Here's how the part is built. I have some questions about the finished solid (model axes, mm). Round coordinates to 2 decimals unless told otherwise and drop trailing zeros. Loops run counter-clockwise (first coordinate to the right, second up) from the corner with the lowest first, then second, coordinate; pieces in that order, holes last. Notation, with made-up numbers: M 10.5,70.5 L 38.5,70.5 A19 ccw 38.5,93.5 Z; hole C -9.5,-27.5 d2. An arc over 180 degrees is marked long. Answer as CSV lines item,"result".
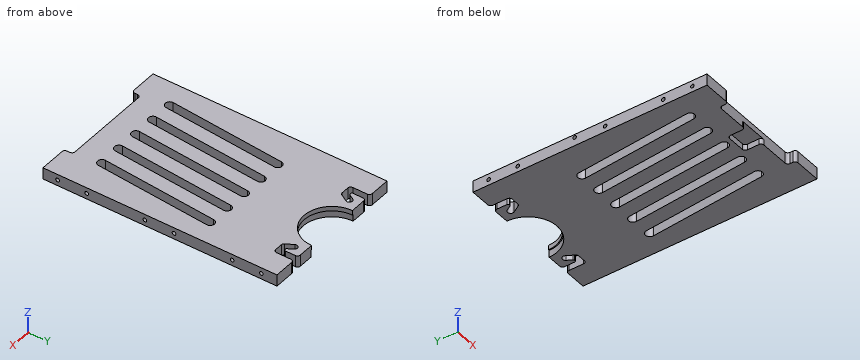
```python
from build123d import *

# Parameters (mm, degrees)
SKETCH1_W                       = 165.1
SKETCH1_H                       = 12.7
BOSS_EXTRUDE1_DEPTH             = 128.5875
SKETCH2_R                       = 30.63494
CUT_EXTRUDE1_DEPTH              = 154.33146336
SKETCH3_R                       = 31.75
CUT_EXTRUDE2_DEPTH              = 7.62
CUT_EXTRUDE3_DEPTH              = 154.33146336
FILLET1_R                       = 3.175
FILLET2_R                       = 1.5875
SKETCH5_W                       = 101.6
SKETCH5_H                       = 9.525
CUT_EXTRUDE4_DEPTH              = 154.33146336
FILLET3_R                       = 3.175
F_21_0_159_DIAMETER_HOLE2_D     = 4.0386
F_21_0_159_DIAMETER_HOLE2_DEPTH = 20.6375
F_21_0_159_DIAMETER_HOLE2_TIP   = 1.213317848
CUT_EXTRUDE5_DEPTH              = 154.33146336
SKETCH11_W                      = 25.4
SKETCH11_H                      = 19.05
CUT_EXTRUDE6_DEPTH              = 6.35
FILLET4_R                       = 3.175


# Read off the part's stored shape, not the designer's step: #21 (0.159) Diameter Hole1
with BuildPart() as part:
    # Sketch1 → Boss-Extrude1 (new, symmetric)
    with BuildSketch(Plane(origin=(0, 0, 0), x_dir=(1, 0, 0), z_dir=(0, 1, 0))):
        Rectangle(SKETCH1_W, SKETCH1_H)
    extrude(amount=BOSS_EXTRUDE1_DEPTH, both=True)

    # Sketch2 → Cut-Extrude1 (cut, through all)
    with BuildSketch(Plane.XY.offset(6.35)):
        with Locations((0, 128.5875)):
            Circle(SKETCH2_R)
    extrude(amount=-CUT_EXTRUDE1_DEPTH, mode=Mode.SUBTRACT)

    # Sketch3 → Cut-Extrude2 (cut)
    with BuildSketch(Plane(origin=(0, 0, -6.35), x_dir=(-1, 0, 0), z_dir=(0, 0, -1))):
        with Locations((0, 128.5875)):
            Circle(SKETCH3_R)
    extrude(amount=-CUT_EXTRUDE2_DEPTH, mode=Mode.SUBTRACT)

    # Sketch4 → Cut-Extrude3 (cut, through all)
    with BuildSketch(Plane.XY.offset(6.35)):
        with BuildLine():
            Line((57.277, 128.5875), (57.277, 106.3625))
            Line((57.277, 106.3625), (43.877983689, 106.3625))
            Line((43.877983689, 106.3625), (38.415384653, 115.823999072))
            ThreePointArc((38.415384653, 115.823999072), (39.623999536, 120.334615615), (44.134615883, 119.126))
            Line((44.134615883, 119.126), (47.690804866, 112.9665))
            Line((47.690804866, 112.9665), (50.673, 112.9665))
            Line((50.673, 112.9665), (50.673, 128.5875))
            Line((50.673, 128.5875), (57.277, 128.5875))
        make_face()
        with BuildLine():
            Line((-50.673, 128.5875), (-57.277, 128.5875))
            Line((-57.277, 128.5875), (-57.277, 106.3625))
            Line((-57.277, 106.3625), (-43.877983689, 106.3625))
            Line((-43.877983689, 106.3625), (-38.415384653, 115.823999072))
            ThreePointArc((-38.415384653, 115.823999072), (-39.623999536, 120.334615615), (-44.134615883, 119.126))
            Line((-44.134615883, 119.126), (-47.690804866, 112.9665))
            Line((-47.690804866, 112.9665), (-50.673, 112.9665))
            Line((-50.673, 112.9665), (-50.673, 128.5875))
        make_face()
    extrude(amount=-CUT_EXTRUDE3_DEPTH, mode=Mode.SUBTRACT)

    # Fillet1
    fillet1_edges = [part.edges().sort_by_distance(p)[0] for p in [
        (50.673, 128.5875, 0),
        (57.277, 128.5875, 0),
        (57.277, 106.3625, 0),
        (43.877983689, 106.3625, 0),
        (-43.877983689, 106.3625, 0),
        (-57.277, 106.3625, 0),
        (-57.277, 128.5875, 0),
        (-50.673, 128.5875, 0),
    ]]
    fillet(fillet1_edges, radius=FILLET1_R)

    # Fillet2
    fillet2_edges = [part.edges().sort_by_distance(p)[0] for p in [
        (47.690804866, 112.9665, 0),
        (50.673, 112.9665, 0),
        (-50.673, 112.9665, 0),
        (-47.690804866, 112.9665, 0),
    ]]
    fillet(fillet2_edges, radius=FILLET2_R)

    # Sketch5 → Cut-Extrude4 (cut, through all)
    with BuildSketch(Plane.XY.offset(6.35)):
        with Locations((0, -123.825)):
            Rectangle(SKETCH5_W, SKETCH5_H)
    extrude(amount=-CUT_EXTRUDE4_DEPTH, mode=Mode.SUBTRACT)

    # Fillet3
    fillet3_edges = [part.edges().sort_by_distance(p)[0] for p in [
        (-50.8, -128.5875, 0),
        (-50.8, -119.0625, 0),
        (50.8, -119.0625, 0),
        (50.8, -128.5875, 0),
    ]]
    fillet(fillet3_edges, radius=FILLET3_R)

    # #21 (0.159) Diameter Hole1 outline → #21 (0.159) Diameter Hole1 (revolve, cut)
    with BuildSketch(Plane(origin=(0, 111.41250006, 0), x_dir=(0, 1, 0), z_dir=(0, 0, -1))):
        Polygon((0, 82.55), (0, 60.699182152), (2.0193, 61.9125), (2.0193, 82.55), align=None)
    revolve(axis=Axis((0, 111.41250006, 0), (1, 0, 0)), mode=Mode.SUBTRACT)

    # 21 _0.159_ Diameter Hole1 2 outline → 21 _0.159_ Diameter Hole1 2 (revolve, cut)
    with BuildSketch(Plane(origin=(0, 79.412500052, 0), x_dir=(0, 1, 0), z_dir=(0, 0, -1))):
        Polygon((0, 82.55), (0, 60.699182152), (2.0193, 61.9125), (2.0193, 82.55), align=None)
    revolve(axis=Axis((0, 79.412500052, 0), (1, 0, 0)), mode=Mode.SUBTRACT)

    # 21 _0.159_ Diameter Hole1 3 outline → 21 _0.159_ Diameter Hole1 3 (revolve, cut)
    with BuildSketch(Plane(origin=(0, 15.412500036, 0), x_dir=(0, 1, 0), z_dir=(0, 0, -1))):
        Polygon((0, 82.55), (0, 60.699182152), (2.0193, 61.9125), (2.0193, 82.55), align=None)
    revolve(axis=Axis((0, 15.412500036, 0), (1, 0, 0)), mode=Mode.SUBTRACT)

    # 21 _0.159_ Diameter Hole1 4 outline → 21 _0.159_ Diameter Hole1 4 (revolve, cut)
    with BuildSketch(Plane(origin=(0, -16.587499972, 0), x_dir=(0, 1, 0), z_dir=(0, 0, -1))):
        Polygon((0, 82.55), (0, 60.699182152), (2.0193, 61.9125), (2.0193, 82.55), align=None)
    revolve(axis=Axis((0, -16.587499972, 0), (1, 0, 0)), mode=Mode.SUBTRACT)

    # 21 _0.159_ Diameter Hole1 5 outline → 21 _0.159_ Diameter Hole1 5 (revolve, cut)
    with BuildSketch(Plane(origin=(0, -80.587499988, 0), x_dir=(0, 1, 0), z_dir=(0, 0, -1))):
        Polygon((0, 82.55), (0, 60.699182152), (2.0193, 61.9125), (2.0193, 82.55), align=None)
    revolve(axis=Axis((0, -80.587499988, 0), (1, 0, 0)), mode=Mode.SUBTRACT)

    # 21 _0.159_ Diameter Hole1 6 outline → 21 _0.159_ Diameter Hole1 6 (revolve, cut)
    with BuildSketch(Plane(origin=(0, -112.587499996, 0), x_dir=(0, 1, 0), z_dir=(0, 0, -1))):
        Polygon((0, 82.55), (0, 60.699182152), (2.0193, 61.9125), (2.0193, 82.55), align=None)
    revolve(axis=Axis((0, -112.587499996, 0), (1, 0, 0)), mode=Mode.SUBTRACT)

    # #21 (0.159) Diameter Hole2
    with Locations(Plane.ZY.offset(82.55)):
        with Locations((0, -112.587499996), (0, -80.587499988), (0, -16.587499972), (2.943873534, 16.784159444), (0, 79.412500052), (0, 111.41250006)):
            Hole(F_21_0_159_DIAMETER_HOLE2_D / 2, depth=F_21_0_159_DIAMETER_HOLE2_DEPTH)
            with Locations((0, 0, -(F_21_0_159_DIAMETER_HOLE2_DEPTH + F_21_0_159_DIAMETER_HOLE2_TIP / 2))):  # 118° drill point
                Cone(0, F_21_0_159_DIAMETER_HOLE2_D / 2, F_21_0_159_DIAMETER_HOLE2_TIP, mode=Mode.SUBTRACT)

    # Sketch10 → Cut-Extrude5 (cut, through all)
    with BuildSketch(Plane.XY.offset(6.35)):
        with BuildLine():
            Line((-60.30687725, -90.072420775), (-49.195816982, 36.927579225))
            ThreePointArc((-49.195816982, 36.927579225), (-44.036360507, 41.25687725), (-39.707062483, 36.097420775))
            Line((-39.707062483, 36.097420775), (-50.81812275, -90.902579225))
            ThreePointArc((-50.81812275, -90.902579225), (-55.977579225, -95.23187725), (-60.30687725, -90.072420775))
        make_face()
        with BuildLine():
            Line((-25.41812275, -90.902579225), (-14.307062483, 36.097420775))
            ThreePointArc((-14.307062483, 36.097420775), (-18.636360507, 41.25687725), (-23.795816982, 36.927579225))
            Line((-23.795816982, 36.927579225), (-34.90687725, -90.072420775))
            ThreePointArc((-34.90687725, -90.072420775), (-30.577579225, -95.23187725), (-25.41812275, -90.902579225))
        make_face()
        with BuildLine():
            Line((-0.01812275, -90.902579225), (11.092937517, 36.097420775))
            ThreePointArc((11.092937517, 36.097420775), (6.763639493, 41.25687725), (1.604183018, 36.927579225))
            Line((1.604183018, 36.927579225), (-9.50687725, -90.072420775))
            ThreePointArc((-9.50687725, -90.072420775), (-5.177579225, -95.23187725), (-0.01812275, -90.902579225))
        make_face()
        with BuildLine():
            Line((25.38187725, -90.902579225), (36.492937517, 36.097420775))
            ThreePointArc((36.492937517, 36.097420775), (32.163639493, 41.25687725), (27.004183018, 36.927579225))
            Line((27.004183018, 36.927579225), (15.89312275, -90.072420775))
            ThreePointArc((15.89312275, -90.072420775), (20.222420775, -95.23187725), (25.38187725, -90.902579225))
        make_face()
        with BuildLine():
            Line((50.78187725, -90.902579225), (61.892937517, 36.097420775))
            ThreePointArc((61.892937517, 36.097420775), (57.563639493, 41.25687725), (52.404183018, 36.927579225))
            Line((52.404183018, 36.927579225), (41.29312275, -90.072420775))
            ThreePointArc((41.29312275, -90.072420775), (45.622420775, -95.23187725), (50.78187725, -90.902579225))
        make_face()
    extrude(amount=-CUT_EXTRUDE5_DEPTH, mode=Mode.SUBTRACT)

    # Sketch11 → Cut-Extrude6 (cut)
    with BuildSketch(Plane(origin=(0, 0, -6.35), x_dir=(-1, 0, 0), z_dir=(0, 0, -1))):
        with Locations((0, -109.5375)):
            Rectangle(SKETCH11_W, SKETCH11_H)
    extrude(amount=-CUT_EXTRUDE6_DEPTH, mode=Mode.SUBTRACT)

    # Fillet4
    fillet4_edges = [part.edges().sort_by_distance(p)[0] for p in [
        (12.7, -119.0625, -3.175),
        (12.7, -100.0125, -3.175),
        (-12.7, -100.0125, -3.175),
        (-12.7, -119.0625, -3.175),
    ]]
    fillet(fillet4_edges, radius=FILLET4_R)


solid = part.part
```
1. For P1, Ø3, axis at y = 111.41, z = 0, coming from the -X side; P2, Ø2.5, axis at y = 79.41, z = 0, coming from the +X side; P3, Ø5, axis at x = 0, z = -0.5, coming from the +Y side, each with a flat end and sliding along its axis, tell me the tip position at first contact or that it passes through.
Evaluation:
P1,"stops at x = -61.6"
P2,"stops at x = 61.45"
P3,"stops at y = 98"
2. I want a section at A-A, the plane x = 69. Please give me the cut outline in (y, z).
Evaluation:
outline,"M -128.59,-6.35 L 128.59,-6.35 L 128.59,6.35 L -128.59,6.35 Z; hole C -112.59,0 d4.04; hole C -80.59,0 d4.04; hole C -16.59,0 d4.04; hole C 15.41,0 d4.04; hole C 79.41,0 d4.04; hole C 111.41,0 d4.04"
3. If I drill on line 1 (Y direction, x = -77, z = 0); line 2 (X direction, y = 27, z = 0.75); line 3 (X direction, y = -28, z = -5), over which ranges is the centre line in solid material (lowest first)? Write a range as [from, to].
Evaluation:
line 1,"y = [-128.59, -114.61], [-110.57, -82.61], [-78.57, -18.61], [-14.57, 77.39], [81.43, 109.39], [113.43, 128.59]"
line 2,"x = [-82.55, -50.06], [-40.5, -24.66], [-15.1, 0.74], [10.3, 26.14], [35.7, 51.54], [61.1, 82.55]"
line 3,"x = [-82.55, -54.88], [-45.31, -29.48], [-19.91, -4.08], [5.49, 21.32], [30.89, 46.72], [56.29, 82.55]"
